Here's how the part is built. I have some questions about the finished solid (model axes, mm). A direction names the side the tool comes from. Round coordinates to 2 decimals unless told otherwise and drop trailing zeros. Write each loop counter-clockwise with the first axis right and the second up, starting at its lowest first coordinate (ties: lowest second). Pieces come first, ordered by that corner, then holes. Notation, with made-up numbers: (36.25, 29.25) -> (55.25, 29.25) arc R30 ccw to (55.25, 51.25) -> close; hole circle Ø8 at (-6.75, 82.25). An arc over 180 degrees is marked (long way). Answer in a Markdown table with one row per item.
from build123d import *

# Parameters (mm, degrees)
SKETCH1_R           = 3
BOSS_EXTRUDE1_DEPTH = 10
BOSS_EXTRUDE2_START = 5
SKETCH1_3_R         = 1.5
BOSS_EXTRUDE2_DEPTH = 2


with BuildPart() as part:
    # Sketch1 → Boss-Extrude1 (new body)
    with BuildSketch(Plane(origin=(0, 0, 0), x_dir=(1, 0, 0), z_dir=(0, 1, 0))):
        with Locations((-5, 2)):
            Circle(SKETCH1_R)
    extrude(amount=BOSS_EXTRUDE1_DEPTH)

    # Sketch1_3 → Boss-Extrude2 (add)
    with BuildSketch(Plane(origin=(0, 0, 0), x_dir=(1, 0, 0), z_dir=(0, 1, 0)).offset(BOSS_EXTRUDE2_START)):
        with BuildLine():
            ThreePointArc((-2.604511851, 0.193999854), (-6.702483219, -0.470131755), (-7.54030513, 3.595885286))
            Line((-7.54030513, 3.595885286), (-10.599067222, -1.273004164))
            ThreePointArc((-10.599067222, -1.273004164), (-9.599794928, -5.584355236), (-5.288443855, -4.585082942))
            Line((-5.288443855, -4.585082942), (-2.604511851, 0.193999854))
        make_face()
        with Locations((-7.943755539, -2.929043553)):
            Circle(SKETCH1_3_R, mode=Mode.SUBTRACT)
        with BuildLine():
            Line((-10.230926638, 7.234880355), (-7.54030513, 3.595885286))
            ThreePointArc((-7.54030513, 3.595885286), (-5.08812745, 4.998705313), (-2.557799528, 3.74231365))
            Line((-2.557799528, 3.74231365), (-6.192479387, 8.837043218))
            ThreePointArc((-6.192479387, 8.837043218), (-9.012784444, 10.055185412), (-10.230926638, 7.234880355))
        make_face()
        with Locations((-8.211703012, 8.035961786)):
            Circle(SKETCH1_3_R, mode=Mode.SUBTRACT)
    extrude(amount=BOSS_EXTRUDE2_DEPTH)


solid = part.part
1) For pin 1 (2 mm diameter, centred on y = 2.5, z = -3.5, fed in from +X); pin 2 (1.5 mm diameter, centred on x = -8, y = 1.5, fed in from +Z); pin 3 (1 mm diameter, centred on x = -7, y = 8, fed in from +Z), each with a flat end and sliding along its axis, tell me the tip position at first contact or that it passes through.
Response:
| item | result |
|---|---|
| pin 1 | stops at x = -2.04 |
| pin 2 | stops at z = -0.02 |
| pin 3 | stops at z = 0.6 |
2) I want a section at A-A, the plane z = 3.75. List the corners of the cut face in (x, y) for me.
Response:
| item | result |
|---|---|
| outline | (-10.96, 5) -> (-9.2, 5) -> (-9.2, 7) -> (-10.96, 7) -> close; (-6.69, 5) -> (-4.82, 5) -> (-4.82, 7) -> (-6.69, 7) -> close |
3) Which directions (+Z, -Z, +X, -X, +Y, -Y) give clear straight access to the entire face, cutting with the end or side of a thin tool? Please do faces 1 (the face through (-2.14, 4.93, -2.9)), 2 (the face through (-5, 0, -2)), 3 (the face through (-8.904, 5.986, -5.441)).
Response:
| item | result |
|---|---|
| face 1 | none |
| face 2 | +Z, -Z, +X, -X, -Y |
| face 3 | -X, +Y, -Y |
4) We'd pull the mould along Z, two halves only. Please class faces 4 (the face through (-8, 7, 1)), 5 (the face through (-9.658, 5.986, 5.547)), 6 (the face through (-9.048, 5.986, -1.196)): +Z half, -Z half, draft (parallel to the pull), parting line (faces both ways), or undercut.
Response:
| item | result |
|---|---|
| face 4 | draft |
| face 5 | parting line |
| face 6 | undercut |
5) I want a section at B-B, the plane y = 6. List the corners of the cut face in (x, z) for me.
Response:
| item | result |
|---|---|
| outline | (-10.6, 1.27) -> (-7.54, -3.6) -> (-10.23, -7.23) arc R2.17 ccw to (-6.19, -8.84) -> (-2.56, -3.74) arc R3 ccw to (-2.6, -0.19) -> (-5.29, 4.59) arc R3.13 ccw to start; hole circle Ø3 at (-8.21, -8.04); hole circle Ø3 at (-7.94, 2.93) |
6) I need wall thicknesses on line 1 (Z direction, x = -5, y = 2); line 2 (Y direction, x = -8.25, z = 0.5); line 3 (X direction, y = 5.5, z = -8). Which ranges of each line are inside material? Lowest first, please. Write a range as [from, to].
Response:
| item | result |
|---|---|
| line 1 | z = [-5, 1] |
| line 2 | y = [5, 7] |
| line 3 | x = [-10.38, -9.71], [-6.71, -5.6] |
7) I want a section at C-C, the plane x = -5. List the corners of the cut face in (y, z) for me, and give its area (3 significant figures).
Response:
| item | result |
|---|---|
| outline | (0, -5) -> (5, -5) -> (5, -7.17) -> (7, -7.17) -> (7, -5) -> (10, -5) -> (10, 1) -> (7, 1) -> (7, 4.07) -> (5, 4.07) -> (5, 1) -> (0, 1) -> close |
| area | 70.5 mm^2 |
